Can you work these out from the model? Positions are in its coordinate system, mm. Face numbers are marked on the shaded views. A direction names the side the tool comes from. Round coordinates to 2 decimals unless told otherwise and drop trailing zeros. Use a Markdown table: item, result.
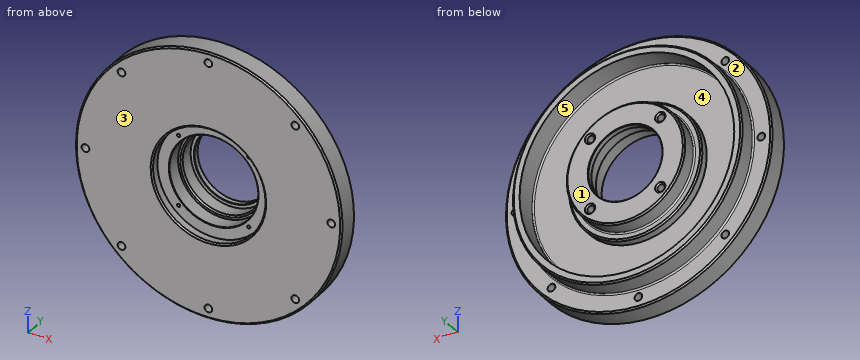
from build123d import *

# Parameters (mm, degrees)
SKETCH_1_R                           = 90
EXTRUDE_1_DEPTH                      = 30
CHAMFER_1_SIZE                       = 1
CHAMFER_3_SIZE                       = 1
CHAMFER_4_SIZE                       = 0.3
FILLET_1_R                           = 1
SKETCH_4_R                           = 1.1
CUT_EXTRUDE_1_DEPTH                  = 131.766968306
CUT_EXTRUDE_START                    = 11
SKETCH_4_3_R                         = 2.5
CUT_EXTRUDE_2_DEPTH                  = 120.766968306
CUT_EXTRUDE_START_2                  = 9
SKETCH_4_4_R                         = 1.1
CUT_EXTRUDE_3_DEPTH                  = 2
CHAMFER_5_SIZE                       = 1
PATTERN_CIRCULAR_1_COUNT             = 4
CHAMFER_5_OF_PATTERN_CIRCULAR_1_SIZE = 1
SKETCH_5_R                           = 2.6
CUT_EXTRUDE_4_DEPTH                  = 131.766968306


with BuildPart() as part:
    # Sketch 1 → Extrude 1 (new body)
    with BuildSketch(Plane(origin=(0, 0, 0), x_dir=(1, 0, 0), z_dir=(0, 1, 0))):
        with Locations(Location((0, 0, 0), (0, 0, 270))):
            Circle(SKETCH_1_R)
    extrude(amount=EXTRUDE_1_DEPTH)

    # Sketch 2 → Cut-Revolve 1 (revolve, cut)
    with BuildSketch(Plane(origin=(0, 0, 0), x_dir=(0, 0, -1), z_dir=(1, 0, 0))):
        Polygon((0, 67.414866474), (0, 0), (-38, 0), (-38, 6), (-30, 6), (-30, 16), (-27.5, 16), (-27.5, 26), (-25, 26), (-25, 67.414866474), align=None)
    revolve(axis=Axis((0, 67.414866474, 0), (0, -1, 0)), mode=Mode.SUBTRACT)

    # Sketch 3 → Cut-Revolve 2 (revolve, cut)
    with BuildSketch(Plane(origin=(0, 0, 0), x_dir=(0, 0, -1), z_dir=(1, 0, 0)), mode=Mode.PRIVATE) as cut_revolve_2_sk:
        Polygon((0, 53.537203253), (0, 30), (-40, 30), (-40, 19), (-45, 19), (-45, 13), (-72.5, 13), (-72.5, 28), (-77.5, 28), (-77.5, 15), (-112.622574603, 15), (-112.622574603, 53.537203253), align=None)
    revolve(cut_revolve_2_sk.sketch.rotate(Axis((0, 0, 0), (0, 1, 0)), 180), axis=Axis((0, 0, 0), (0, 1, 0)), mode=Mode.SUBTRACT)

    # Chamfer 1
    chamfer_1_edges = [part.edges().sort_by_distance(p)[0] for p in [
        (0, 19, 45),
        (0, 16, -27.5),
    ]]
    chamfer(chamfer_1_edges, length=CHAMFER_1_SIZE)

    # Chamfer 3
    chamfer_3_edges = [part.edges().sort_by_distance(p)[0] for p in [
        (0, 15, -90),
        (0, 28, 77.5),
        (0, 30, 40),
        (0, 0, -90),
        (0, 0, -38),
    ]]
    chamfer(chamfer_3_edges, length=CHAMFER_3_SIZE)

    # Chamfer 4
    chamfer_4_edges = [part.edges().sort_by_distance(p)[0] for p in [
        (0, 30, -25),
        (0, 26, -25),
        (0, 6, -30),
    ]]
    chamfer(chamfer_4_edges, length=CHAMFER_4_SIZE)

    # Fillet 1
    fillet_1_edges = [part.edges().sort_by_distance(p)[0] for p in [
        (0, 15, 77.5),
        (0, 13, 72.5),
        (0, 19, 40),
    ]]
    fillet(fillet_1_edges, radius=FILLET_1_R)

    # Sketch 4 → Cut-Extrude 1 (cut, through all)
    with BuildSketch(Plane(origin=(0, 0, 0), x_dir=(1, 0, 0), z_dir=(0, 1, 0))):
        with Locations(Location((23.68807717, 23.68807717, 0), (0, 0, 90))):
            Circle(SKETCH_4_R)
    cut_extrude_1 = extrude(amount=CUT_EXTRUDE_1_DEPTH, mode=Mode.SUBTRACT)

    # Sketch 4_3 → Cut-Extrude 2 (cut, through all)
    with BuildSketch(Plane(origin=(0, 0, 0), x_dir=(1, 0, 0), z_dir=(0, 1, 0)).offset(CUT_EXTRUDE_START)):
        with Locations(Location((23.68807717, 23.68807717, 0), (0, 0, 270))):
            Circle(SKETCH_4_3_R)
    cut_extrude_2 = extrude(amount=CUT_EXTRUDE_2_DEPTH, mode=Mode.SUBTRACT)

    # Sketch 4_4 → Cut-Extrude 3 (cut)
    with BuildSketch(Plane(origin=(0, 0, 0), x_dir=(1, 0, 0), z_dir=(0, 1, 0)).offset(CUT_EXTRUDE_START_2)):
        Polygon((21.401599273, 23.075417264), (23.075417264, 21.401599273), (25.361895161, 22.014259179), (25.974555067, 24.300737076), (24.300737076, 25.974555067), (22.014259179, 25.361895161), align=None)
        with Locations(Location((23.68807717, 23.68807717, 0), (0, 0, 90))):
            Circle(SKETCH_4_4_R, mode=Mode.SUBTRACT)
    cut_extrude_3 = extrude(amount=CUT_EXTRUDE_3_DEPTH, mode=Mode.SUBTRACT)

    # Chamfer 5
    chamfer_5_edges = [part.edges().sort_by_distance(p)[0] for p in [
        (23.68807717, 30, -26.18807717),
    ]]
    chamfer(chamfer_5_edges, length=CHAMFER_5_SIZE)

    # Pattern Circular 1: Cut-Extrude 1, Cut-Extrude 2, Cut-Extrude 3 ×4 about axis
    pattern_circular_1_axis = Axis((0, 0, 0), (0, 1, 0))
    add([cut_extrude_1.rotate(pattern_circular_1_axis, i * 360 / PATTERN_CIRCULAR_1_COUNT) for i in range(1, PATTERN_CIRCULAR_1_COUNT)], mode=Mode.SUBTRACT)
    add([cut_extrude_2.rotate(pattern_circular_1_axis, i * 360 / PATTERN_CIRCULAR_1_COUNT) for i in range(1, PATTERN_CIRCULAR_1_COUNT)], mode=Mode.SUBTRACT)
    add([cut_extrude_3.rotate(pattern_circular_1_axis, i * 360 / PATTERN_CIRCULAR_1_COUNT) for i in range(1, PATTERN_CIRCULAR_1_COUNT)], mode=Mode.SUBTRACT)

    # Chamfer 5 of Pattern Circular 1
    chamfer_5_of_pattern_circular_1_edges = [part.edges().sort_by_distance(p)[0] for p in [
        (-26.18807717, 30, -23.68807717),
        (-23.68807717, 30, 26.18807717),
        (26.18807717, 30, 23.68807717),
    ]]
    chamfer(chamfer_5_of_pattern_circular_1_edges, length=CHAMFER_5_OF_PATTERN_CIRCULAR_1_SIZE)

    # Sketch 5 → Cut-Extrude 4 (cut, through all)
    with BuildSketch(Plane(origin=(0, 0, 0), x_dir=(1, 0, 0), z_dir=(0, 1, 0))):
        with Locations(Location((83, 0, 0), (0, 0, 90))):
            Circle(SKETCH_5_R)
        with Locations(Location((58.689862838, -58.689862838, 0), (0, 0, 90))):
            Circle(SKETCH_5_R)
        with Locations(Location((0, -83, 0), (0, 0, 90))):
            Circle(SKETCH_5_R)
        with Locations(Location((-58.689862838, -58.689862838, 0), (0, 0, 90))):
            Circle(SKETCH_5_R)
        with Locations(Location((-83, 0, 0), (0, 0, 90))):
            Circle(SKETCH_5_R)
        with Locations(Location((-58.689862838, 58.689862838, 0), (0, 0, 90))):
            Circle(SKETCH_5_R)
        with Locations(Location((0, 83, 0), (0, 0, 90))):
            Circle(SKETCH_5_R)
        with Locations(Location((58.689862838, 58.689862838, 0), (0, 0, 90))):
            Circle(SKETCH_5_R)
    extrude(amount=CUT_EXTRUDE_4_DEPTH, mode=Mode.SUBTRACT)


solid = part.part
1. Will these pins go through, and if not, where does the flat tip stop? pin 1 Ø10 at (x, z) = (18.5, -51) entering from +Y; pin 2 Ø10 at (x, z) = (-56.5, 43) entering from +Y; pin 3 Ø2 at (x, y) = (-2, 21.5) entering from -Z.
Answer sheet:
| item | result |
|---|---|
| pin 1 | stops at y = 13 |
| pin 2 | stops at y = 28 |
| pin 3 | stops at z = -77.49 |
2. Which directions (+Z, -Z, +X, -X, +Y, -Y) give clear straight access to the entire face, cutting with the end or side of a thin tool? Please do the marked faces 1 and 2.
Answer sheet:
| item | result |
|---|---|
| face 1 | +Z, -Z, +X, -X, +Y |
| face 2 | +Y |
3. I want a section at A-A (x = 0). State how many separate pieces and enclosed holes the cut face has, plus the area to 3 significant figures.
Answer sheet:
| item | result |
|---|---|
| separate pieces | 4 |
| enclosed holes | 0 |
| area | 1,990 mm² |
4. I need wall thicknesses on line 1 (Z direction, x = 1, y = 18); line 2 (X direction, y = 23.5, z = 0); line 3 (X direction, y = 9.5, z = 0). Which ranges of each line are inside material? Lowest first, please.
Answer sheet:
| item | result |
|---|---|
| line 1 | z = -77.49 to -72.49, -44.99 to -27.48, 27.48 to 44.99, 72.49 to 77.49 |
| line 2 | x = -77.5 to -72.5, -40 to -27.5, 27.5 to 40, 72.5 to 77.5 |
| line 3 | x = -90 to -85.6, -80.4 to -30, 30 to 80.4, 85.6 to 90 |
5. If we mould it in two halves opening along Z, with no side actions, what happens to the marked faces 3, 4 and 5? For each: +Z half, -Z half, draft (parallel to the pull), parting line (faces both ways), or undercut.
Answer sheet:
| item | result |
|---|---|
| face 3 | draft |
| face 4 | undercut |
| face 5 | undercut |
